```python
from build123d import *

# Parameters (mm, degrees)
SKETCH1_W               = 13.1
SKETCH1_H               = 5.8
BOSS_EXTRUDE1_DEPTH     = 5
SKETCH10_W              = 5.65
SKETCH10_H              = 4.6
CUT_EXTRUDE7_DEPTH      = 6.6
SKETCH9_R               = 0.75
CUT_EXTRUDE6_DEPTH      = 6
CUT_EXTRUDE6_DEPTH_BACK = 6


with BuildPart() as part:
    # Sketch1 → Boss-Extrude1 (new body, symmetric)
    with BuildSketch(Plane(origin=(0, 0, 0), x_dir=(1, 0, 0), z_dir=(0, 1, 0))):
        Rectangle(SKETCH1_W, SKETCH1_H)
    extrude(amount=BOSS_EXTRUDE1_DEPTH, both=True)

    # Sketch10 → Cut-Extrude7 (cut)
    with BuildSketch(Plane(origin=(0, 5, 0), x_dir=(1, 0, 0), z_dir=(0, 1, 0))):
        with Locations((-3.125, 0)):
            Rectangle(SKETCH10_W, SKETCH10_H)
        with Locations((3.125, 0)):
            Rectangle(SKETCH10_W, SKETCH10_H)
    extrude(amount=-CUT_EXTRUDE7_DEPTH, mode=Mode.SUBTRACT)

    # Sketch9 → Cut-Extrude6 (cut, two sides)
    with BuildSketch(Plane(origin=(0, 0, 0), x_dir=(1, 0, 0), z_dir=(0, 1, 0))) as cut_extrude6_sk:
        with Locations((-4.625, 0)):
            Circle(SKETCH9_R)
        with Locations((-1.625, 0)):
            Circle(SKETCH9_R)
        with Locations((1.625, 0)):
            Circle(SKETCH9_R)
        with Locations((4.625, 0)):
            Circle(SKETCH9_R)
    extrude(amount=CUT_EXTRUDE6_DEPTH, mode=Mode.SUBTRACT)
    extrude(cut_extrude6_sk.sketch, amount=-CUT_EXTRUDE6_DEPTH_BACK, mode=Mode.SUBTRACT)


solid = part.part
```
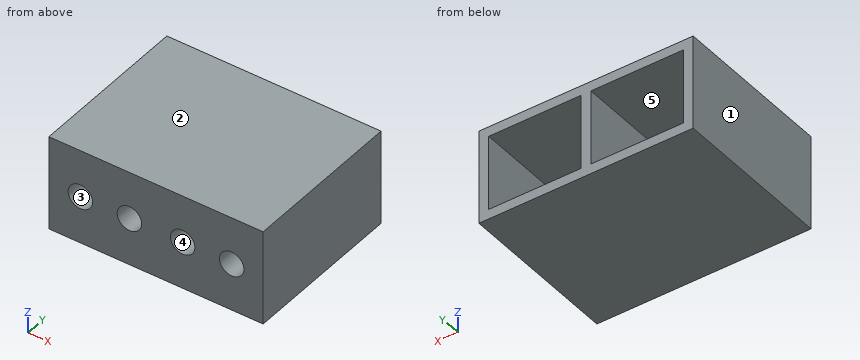
For this review, take the finished solid that the model builds, in its own axes (mm). Face numbers are marked on the shaded views. A direction names the side the tool comes from. Give positions to 0.01 mm unless a question says otherwise; leave off trailing zeros. Write each loop counter-clockwise with the first axis right and the second up, starting at its lowest first coordinate (ties: lowest second). Pieces come first, ordered by that corner, then holes. Notation, with made-up numbers: M 3,82 L 18,82 A24 cw 18,94 Z; hole C -36.5,52.25 d5. An arc over 180 degrees is marked long. Answer as CSV lines item,"result".
1. For the marked faces 4 and 5, list the 3-axis set-ups (+Z, -Z, +X, -X, +Y, -Y) from which the entire face can be reached by the end or side of a thin tool; tool diameter is ignored.
Findings:
face 4,"+Y, -Y"
face 5,"+Y"
2. For pin 1 (1.7 mm diameter, centred on x = 4.625, z = 0, fed in from +Y); pin 2 (1.2 mm diameter, centred on x = -1.625, z = 0, fed in from +Y), all flat-tipped, find the tip position at first contact; note any pin that passes through.
Findings:
pin 1,"stops at y = -1.6"
pin 2,"passes through"
3. Consider section C-C, the plane x = -4.5. Write out the cut boundary in (y, z).
Findings:
outline,"M -5,-2.9 L 5,-2.9 L 5,-2.3 L -1.6,-2.3 L -1.6,-0.74 L -5,-0.74 Z; M -5,0.74 L -1.6,0.74 L -1.6,2.3 L 5,2.3 L 5,2.9 L -5,2.9 Z"
4. Draft analysis for pull direction Z (two halves, no side actions). For the marked faces 1, 2 and 3, state which applies: +Z half, -Z half, draft (parallel to the pull), parting line (faces both ways), or undercut.
Findings:
face 1,"draft"
face 2,"+Z half"
face 3,"undercut"
5. Consider section D-D, the plane y = 4.25. Write out the cut boundary in (x, z), then the cut area to 3 significant figures.
Findings:
outline,"M -6.55,-2.9 L 6.55,-2.9 L 6.55,2.9 L -6.55,2.9 Z; hole M -5.95,-2.3 L -0.3,-2.3 L -0.3,2.3 L -5.95,2.3 Z; hole M 0.3,-2.3 L 5.95,-2.3 L 5.95,2.3 L 0.3,2.3 Z"
area,"24.0 mm2"
6. Consider section A-A, the plane z = 0. Write out the cut boundary in (x, y) (3 decimals), then the cut area to 3 significant figures.
Findings:
outline,"M -6.55,-5 L -5.375,-5 L -5.375,-1.6 L -5.95,-1.6 L -5.95,5 L -6.55,5 Z; M -3.875,-5 L -2.375,-5 L -2.375,-1.6 L -3.875,-1.6 Z; M -0.875,-5 L 0.875,-5 L 0.875,-1.6 L 0.3,-1.6 L 0.3,5 L -0.3,5 L -0.3,-1.6 L -0.875,-1.6 Z; M 2.375,-5 L 3.875,-5 L 3.875,-1.6 L 2.375,-1.6 Z; M 5.375,-5 L 6.55,-5 L 6.55,5 L 5.95,5 L 5.95,-1.6 L 5.375,-1.6 Z"
area,"36.0 mm2"
7. Consider section B-B, the plane y = -3.25. Write out the cut boundary in (x, z) (3 decimals).
Findings:
outline,"M -6.55,-2.9 L 6.55,-2.9 L 6.55,2.9 L -6.55,2.9 Z; hole C -4.625,0 d1.5; hole C -1.625,0 d1.5; hole C 1.625,0 d1.5; hole C 4.625,0 d1.5"
8. Wall thickness on line 1 (X direction, y = 4.25, z = 1.05); line 2 (X direction, y = -2.9, z = 0) (3 decimals); line 3 (Z direction, x = 5.25, y = 1.25): over which ranges is each line inside the solid? List them lowest first.
Findings:
line 1,"x = -6.55 to -5.95, -0.3 to 0.3, 5.95 to 6.55"
line 2,"x = -6.55 to -5.375, -3.875 to -2.375, -0.875 to 0.875, 2.375 to 3.875, 5.375 to 6.55"
line 3,"z = -2.9 to -2.3, 2.3 to 2.9"
